Source: CAD feature listing. Evaluate the final solid. Frame: model axes, mm. Face numbers are marked on the shaded views. A direction names the side the tool comes from. Give positions to 0.01 mm unless a question says otherwise; leave off trailing zeros. Write each loop counter-clockwise with the first axis right and the second up, starting at its lowest first coordinate (ties: lowest second). Pieces come first, ordered by that corner, then holes. Notation, with made-up numbers: M 31,77 L 68,77 A5 cw 68,83 Z; hole C 78.25,34 d1. An arc over 180 degrees is marked long. Answer as a JSON object with one key per item and string values. Group by question number.
```python
from build123d import *

# Parameters (mm, degrees)
ESQUISSE1_W             = 15
ESQUISSE1_H             = 15
EXTRUSION1_DEPTH        = 100
ESQUISSE2_W             = 12
ESQUISSE2_H             = 12
EXTRUSION2_DEPTH        = 101.560926806
CONG_1_R                = 7.5
ESQUISSE3_R             = 1.5
EXTRUSION3_DEPTH        = 102.396498953
ESQUISSE4_W             = 12
ESQUISSE4_H             = 20
ENL_V_MAT_EXTRU_1_DEPTH = 3
CONG_2_R                = 3


with BuildPart() as part:
    # Esquisse1 → Extrusion1 (new body)
    with BuildSketch(Plane.XY):
        Rectangle(ESQUISSE1_W, ESQUISSE1_H)
    extrude(amount=EXTRUSION1_DEPTH)

    # Esquisse2 → Extrusion2 (cut, through all)
    with BuildSketch(Plane.XY.offset(100)):
        Rectangle(ESQUISSE2_W, ESQUISSE2_H)
    extrude(amount=-EXTRUSION2_DEPTH, mode=Mode.SUBTRACT)

    # Congé1
    # the kernel refuses this fillet: 7.5 mm, written as the material it takes off along each edge
    with BuildSketch(Plane(origin=(-26.25, -7.5, 0), x_dir=(0, 0, 1), z_dir=(1, 0, 0))) as cong_1_piece_1:
        with BuildLine():
            CenterArc((CONG_1_R, -CONG_1_R), CONG_1_R, 90, 90)
            Line((0, -CONG_1_R), (0, 0))
            Line((0, 0), (CONG_1_R, 0))
        make_face()
    extrude(amount=52.5, mode=Mode.SUBTRACT)
    with BuildSketch(Plane(origin=(26.25, 7.5, 0), x_dir=(0, -1, 0), z_dir=(-1, 0, 0))) as cong_1_piece_2:
        with BuildLine():
            CenterArc((CONG_1_R, CONG_1_R), CONG_1_R, 180, 90)
            Line((0, CONG_1_R), (0, 0))
            Line((0, 0), (CONG_1_R, 0))
        make_face()
    extrude(amount=52.5, mode=Mode.SUBTRACT)

    # Esquisse3 → Extrusion3 (cut, through all)
    with BuildSketch(Plane(origin=(7.5, 0, 0), x_dir=(0, 0, -1), z_dir=(1, 0, 0))):
        with Locations((-7.5, 0)):
            Circle(ESQUISSE3_R)
    extrude(amount=-EXTRUSION3_DEPTH, mode=Mode.SUBTRACT)

    # Esquisse4 → Enlèv. mat.-Extru.1 (cut)
    with BuildSketch(Plane(origin=(0, 7.5, 0), x_dir=(-1, 0, 0), z_dir=(0, 1, 0))):
        with Locations((0, 32.5)):
            Rectangle(ESQUISSE4_W, ESQUISSE4_H)
    extrude(amount=-ENL_V_MAT_EXTRU_1_DEPTH, mode=Mode.SUBTRACT)

    # Congé2
    cong_2_edges = [part.edges().sort_by_distance(p)[0] for p in [
        (-6, 6.75, 42.5),
        (-6, 6.75, 22.5),
        (6, 6.75, 22.5),
        (6, 6.75, 42.5),
    ]]
    fillet(cong_2_edges, radius=CONG_2_R)


solid = part.part
```
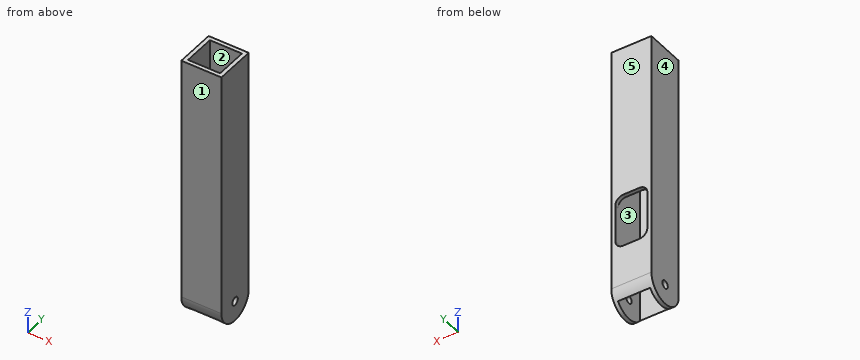
(1) Section A-A, the plane x = -1.75. Return loops of the section in (y, z).
(2) Ray query, L1, parallel to X at y = 0.75, z = 38.5; L2, parallel to Y at x = 6.6, z = 7.5. Return the intervals inside material, ascending. Write a range as [from, to].
(3) Section C-C, the plane z = 65. Return loops of the section in (x, y).
(4) Section B-B, the plane y = 0. Return loops of the section in (x, z), plus the area to 3 significant figures.
(5) Contact query for flat-ended pins moving along their axis: pin 1 Ø0.8 at (x, y) = (-1, 6.5) entering from -Z; pin 2 Ø5 at (y, z) = (0, 7.5) entering from +X. Output: stop coordinate, or through.
(6) Pull-direction query (X, two-part tool) for the marked faces 3, 4 and 5; classes: pulls with the +X half, pulls with the -X half, needs draft (parallel to the pull), parting line crosses it, or undercut.
(7) Access query for the marked faces 1 and 2. Directions: +Z, -Z, +X, -X, +Y, -Y. A direction counts if a zero-diameter tool reaches every point of the face in a straight line with its end or side. Return the directions, or none.
Reported:
{
 "1": {"outline": "M -7.5,7.5 A7.5 ccw -6,3 L -6,100 L -7.5,100 Z; M 6,3 A7.5 ccw 7.5,7.5 L 7.5,22.5 L 6,22.5 Z; M 6,42.5 L 7.5,42.5 L 7.5,100 L 6,100 Z"},
 "2": {"L1": "x = [-7.5, -6], [6, 7.5]", "L2": "y = [-7.5, -1.5], [1.5, 7.5]"},
 "3": {"outline": "M -7.5,-7.5 L 7.5,-7.5 L 7.5,7.5 L -7.5,7.5 Z; hole M -6,-6 L 6,-6 L 6,6 L -6,6 Z"},
 "4": {"outline": "M -7.5,0 L -6,0 L -6,6 L -7.5,6 Z; M -7.5,9 L -6,9 L -6,100 L -7.5,100 Z; M 6,0 L 7.5,0 L 7.5,6 L 6,6 Z; M 6,9 L 7.5,9 L 7.5,100 L 6,100 Z", "area": "291 mm2"},
 "5": {"pin 1": "stops at z = 3.14", "pin 2": "stops at x = 7.5"},
 "6": {"face 3": "undercut", "face 4": "pulls with the -X half", "face 5": "needs draft"},
 "7": {"face 1": "+Z, -Z, +X, -X, -Y", "face 2": "+Z, -Z"}
}
